The model under review builds one solid part; all positions refer to its coordinate system, in mm. Round coordinates to 2 decimals unless told otherwise and drop trailing zeros. Loops run counter-clockwise (first coordinate to the right, second up) from the corner with the lowest first, then second, coordinate; pieces in that order, holes last. Notation, with made-up numbers: (6, -25) -> (49, -25) arc R7 cw to (49, -19) -> close; hole circle Ø5 at (5, 88.5). An arc over 180 degrees is marked (long way). Use a Markdown table: item, result. Add a question column.
1) Consider section B-B on x = 12.7. Give the boundary of the cut face in (y, z), plus the area to 3 significant figures.
2) Insertion check: pin 1 (5.5 mm diameter, centred on x = 53.98, z = 4.76, fed in from +Y); pin 2 (2.5 mm diameter, centred on x = 38.1, y = 51.75, fed in from -Z); pin 3 (8 mm diameter, centred on x = 59.5, y = 49.5, fed in from +Z); pin 4 (1 mm diameter, centred on y = 65.5, z = -1, fed in from -X) (3 decimals). Each pin has a flat end and moves straight along its axis. Give the tip position at first contact, or say it passes through.
3) Consider section D-D on x = 68.6. Give the boundary of the cut face in (y, z).
4) Consider section A-A on y = 4.65. Give the boundary of the cut face in (x, z), plus the area to 3 significant figures.
5) Consider section C-C on z = 19.05. Give the boundary of the cut face in (x, y) (1 decimal).
6) Wall thickness on probe 1 along Y at (x, z) = (38.1, -0.65); probe 2 along Y at (x, z) = (68.6, -1.1); probe 3 along Z at (x, y) = (65.5, 45): over which ranges is each line inside the solid? List them lowest first.
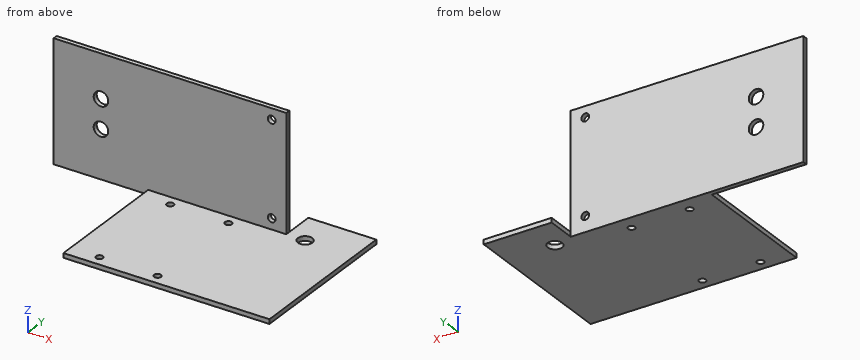
from build123d import *

# Parameters (mm, degrees)
SKETCH1_R           = 3.175
SKETCH1_R_2         = 1.5
BOSS_EXTRUDE1_DEPTH = 2
BOSS_EXTRUDE2_DEPTH = 52.8
SKETCH3_R           = 1.7
SKETCH3_R_2         = 3.175
CUT_EXTRUDE1_DEPTH  = 119.706360402


with BuildPart() as part:
    # Sketch1 → Boss-Extrude1 (new body)
    with BuildSketch(Plane.XY):
        Polygon((0, 58.4), (60.325, 58.4), (60.325, 71.1), (90, 71.1), (90, 58.4), (90, 0), (0, 0), align=None)
        with Locations((68.6, 56.33204182)):
            Circle(SKETCH1_R, mode=Mode.SUBTRACT)
        with Locations((12.7, 51.75)):
            Circle(SKETCH1_R_2, mode=Mode.SUBTRACT)
        with Locations((38.1, 51.75)):
            Circle(SKETCH1_R_2, mode=Mode.SUBTRACT)
        with Locations((12.7, 4.65)):
            Circle(SKETCH1_R_2, mode=Mode.SUBTRACT)
        with Locations((38.1, 4.65)):
            Circle(SKETCH1_R_2, mode=Mode.SUBTRACT)
    extrude(amount=-BOSS_EXTRUDE1_DEPTH)

    # Sketch2 → Boss-Extrude2 (add)
    with BuildSketch(Plane(origin=(0, 0, -2), x_dir=(-1, 0, 0), z_dir=(0, 0, -1))):
        Polygon((0, 56.4), (41.275, 56.4), (41.275, 58.4), (0, 58.4), (-60.325, 58.4), (-60.325, 56.4), align=None)
    extrude(amount=-BOSS_EXTRUDE2_DEPTH)

    # Sketch3 → Cut-Extrude1 (cut, through all)
    with BuildSketch(Plane(origin=(0, 58.4, 0), x_dir=(1, 0, 0), z_dir=(0, 1, 0))):
        with Locations(Location((53.975, -4.7625, 0), (0, 0, 270))):
            Circle(SKETCH3_R)
        with Locations(Location((53.975, -46.0375, 0), (0, 0, 270))):
            Circle(SKETCH3_R)
        with Locations(Location((-20.6375, -31.75, 0), (0, 0, 270))):
            Circle(SKETCH3_R_2)
        with Locations(Location((-20.6375, -19.05, 0), (0, 0, 270))):
            Circle(SKETCH3_R_2)
    extrude(amount=-CUT_EXTRUDE1_DEPTH, mode=Mode.SUBTRACT)


solid = part.part
Result set:
| question | item | result |
|---|---|---|
| 1 | outline | (0, -2) -> (3.15, -2) -> (3.15, 0) -> (0, 0) -> close; (6.15, -2) -> (50.25, -2) -> (50.25, 0) -> (6.15, 0) -> close; (53.25, -2) -> (58.4, -2) -> (58.4, 50.8) -> (56.4, 50.8) -> (56.4, 0) -> (53.25, 0) -> close |
| 1 | area | 206 mm2 |
| 2 | pin 1 | y = 58.4 |
| 2 | pin 2 | through |
| 2 | pin 3 | z = 0 |
| 2 | pin 4 | x = 60.325 |
| 3 | outline | (0, -2) -> (53.16, -2) -> (53.16, 0) -> (0, 0) -> close; (59.51, -2) -> (71.1, -2) -> (71.1, 0) -> (59.51, 0) -> close |
| 4 | outline | (0, -2) -> (11.2, -2) -> (11.2, 0) -> (0, 0) -> close; (14.2, -2) -> (36.6, -2) -> (36.6, 0) -> (14.2, 0) -> close; (39.6, -2) -> (90, -2) -> (90, 0) -> (39.6, 0) -> close |
| 4 | area | 168 mm2 |
| 5 | outline | (-41.3, 56.4) -> (-23.8, 56.4) -> (-23.8, 58.4) -> (-41.3, 58.4) -> close; (-17.5, 56.4) -> (60.3, 56.4) -> (60.3, 58.4) -> (-17.5, 58.4) -> close |
| 6 | probe 1 | 0 to 3.15, 6.15 to 50.25, 53.25 to 58.4 |
| 6 | probe 2 | 0 to 53.16, 59.51 to 71.1 |
| 6 | probe 3 | -2 to 0 |
